CAD build for the part. Positions are in the model's coordinates, mm. Face numbers are marked on the shaded views. A direction names the side the tool comes from. Round coordinates to 2 decimals unless told otherwise and drop trailing zeros. Order: outer loops, then holes, each group sorted by start corner. A loop starts at its lowest first (then second) coordinate and runs counter-clockwise, first axis right, second up.
```python
from build123d import *

# Parameters (mm, degrees)
SKETCH_W        = 165
SKETCH_H        = 45
PAD_DEPTH       = 22
SKETCH001_W     = 133
SKETCH001_H     = 41
POCKET_DEPTH    = 20
SKETCH002_W     = 26
SKETCH002_H     = 41
POCKET001_DEPTH = 20
SKETCH003_W     = 42
SKETCH003_H     = 47
PAD001_DEPTH    = 2
SKETCH008_W     = 42
SKETCH008_H     = 25
PAD002_DEPTH    = 6
SKETCH005_W     = 30
SKETCH005_H     = 13
POCKET002_DEPTH = 8.001
SKETCH009_R     = 1.5
POCKET003_DEPTH = 8.001
SKETCH007_R     = 2.5
POCKET004_DEPTH = 5
SKETCH011_W     = 88.399971
SKETCH011_H     = 21.999902
PAD003_DEPTH    = 2
SKETCH012_W     = 34.60038
SKETCH012_H     = 21.999496
PAD004_DEPTH    = 2


with BuildPart() as part:
    # Sketch → Pad (new body)
    with BuildSketch(Plane.XY):
        with Locations((82.5, 22.5)):
            Rectangle(SKETCH_W, SKETCH_H)
    extrude(amount=PAD_DEPTH)

    # Sketch001 (on Face6 of Pad) → Pocket (cut)
    with BuildSketch(Plane.XY.offset(22)):
        with Locations((68.54825, 22.488898)):
            Rectangle(SKETCH001_W, SKETCH001_H)
    extrude(amount=-POCKET_DEPTH, mode=Mode.SUBTRACT)

    # Sketch002 (on Face5 of Pocket) → Pocket001 (cut)
    with BuildSketch(Plane.XY.offset(22)):
        with Locations((149.979632, 22.458033)):
            Rectangle(SKETCH002_W, SKETCH002_H)
    extrude(amount=-POCKET001_DEPTH, mode=Mode.SUBTRACT)

    # Sketch003 (on Face1 of Pocket001) → Pad001 (join)
    with BuildSketch(Plane(origin=(0, 45, 0), x_dir=(-1, 0, 0), z_dir=(0, 1, 0))):
        with Locations((-55.599999, 23.509954)):
            Rectangle(SKETCH003_W, SKETCH003_H)
    extrude(amount=PAD001_DEPTH)

    # Sketch008 (on Face10 of Pad001) → Pad002 (join)
    with BuildSketch(Plane.XZ.offset(-45)):
        with Locations((55.598549, 34.508675)):
            Rectangle(SKETCH008_W, SKETCH008_H)
    extrude(amount=PAD002_DEPTH)

    # Sketch005 (on Face28 of Pad002) → Pocket002 (cut, through all)
    with BuildSketch(Plane.XZ.offset(-39)):
        with Locations((55.035654, 34.372233)):
            Rectangle(SKETCH005_W, SKETCH005_H)
    extrude(amount=-POCKET002_DEPTH, mode=Mode.SUBTRACT)

    # Sketch009 (on Face32 of Pocket002) → Pocket003 (cut, through all)
    with BuildSketch(Plane.XZ.offset(-39)):
        with Locations((37.021919, 34.390724)):
            Circle(SKETCH009_R)
        with Locations((72.989189, 34.493778)):
            Circle(SKETCH009_R)
    extrude(amount=-POCKET003_DEPTH, mode=Mode.SUBTRACT)

    # Sketch007 (on Face3 of Pocket003) → Pocket004 (cut)
    with BuildSketch(Plane.YZ.offset(165)):
        with Locations((37.952961, 13.56812)):
            Circle(SKETCH007_R)
    extrude(amount=-POCKET004_DEPTH, mode=Mode.SUBTRACT)

    # Sketch011 (on Face2 of Pocket004) → Pad003 (join)
    with BuildSketch(Plane(origin=(0, 45, 0), x_dir=(-1, 0, 0), z_dir=(0, 1, 0))):
        with Locations((-120.799969, 11.000045)):
            Rectangle(SKETCH011_W, SKETCH011_H)
    extrude(amount=PAD003_DEPTH)

    # Sketch012 (on Face2 of Pad003) → Pad004 (join)
    with BuildSketch(Plane(origin=(0, 45, 0), x_dir=(-1, 0, 0), z_dir=(0, 1, 0))):
        with Locations((-17.30019, 10.999748)):
            Rectangle(SKETCH012_W, SKETCH012_H)
    extrude(amount=PAD004_DEPTH)


solid = part.part
```
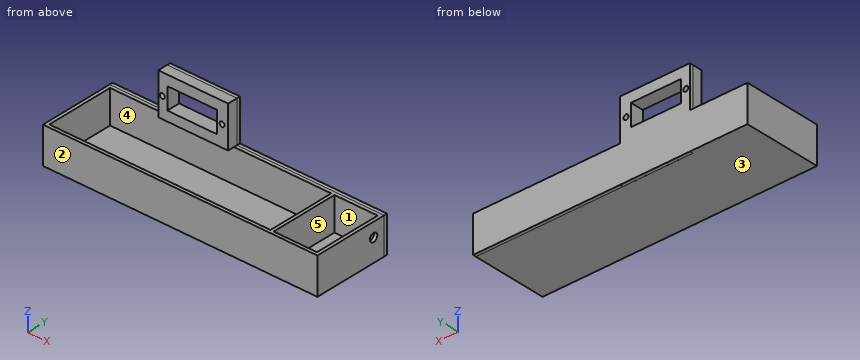
1. Cut at D-D, the plane y = 4. Write the cut outline in (x, z), and give its area (3 significant figures).
2. Cut at A-A, the plane z = 9.5. Give the number of separate pieces and of enclosed holes in the cut face, and give its area (3 significant figures).
3. Cut at C-C, the plane y = 37. Write the cut outline in (x, z).
4. Tool access for the marked faces 1 and 2: list every direction of +Z, -Z, +X, -X, +Y, -Y with a clear straight run to the whole face (end or side of a thin tool).
5. Pin check, flat tips, straight feed: P1, Ø1, axis at y = 46, z = 35, coming from the +X side; P2, Ø5, axis at y = 40.5, z = 33.5, coming from the -X side; P3, Ø20, axis at x = 65, z = 33.5, coming from the -Y side; P4, Ø4, axis at y = 23.5, z = 25, coming from the -X side. Stop position of each tip, or through.
6. Mould opens along Z. For the marked faces 3, 4 and 5 say: released by +Z, released by -Z, zero draft, split by the parting line, or undercut.
7. Drill centre lines: line 1 (X direction, y = 25.5, z = 12); line 2 (Y direction, x = 62, z = 15); line 3 (Z direction, x = 38, y = 40). Where is each one in solid material? Low to high.
Outcome:
1. outline: (0, 0) - (165, 0) - (165, 22) - (162.98, 22) - (162.98, 2) - (136.98, 2) - (136.98, 22) - (135.05, 22) - (135.05, 2) - (2.05, 2) - (2.05, 22) - (0, 22) - close
1. area: 450 mm2
2. separate pieces: 1
2. enclosed holes: 2
2. area: 1,240 mm2
3. outline: (0, 0) - (165, 0) - (165, 11.26) - (162.98, 11.26) - (162.98, 2) - (136.98, 2) - (136.98, 22) - (135.05, 22) - (135.05, 2) - (2.05, 2) - (2.05, 22) - (0, 22) - close; (162.98, 15.88) - (165, 15.88) - (165, 22) - (162.98, 22) - close
4. face 1: +Z
4. face 2: +Z, -Z, +X, -X, -Y
5. P1: stops at x = 76.6
5. P2: stops at x = 34.6
5. P3: stops at y = 39
5. P4: passes through
6. face 3: released by -Z
6. face 4: undercut
6. face 5: zero draft
7. line 1: x = 0 to 2.05, 135.05 to 136.98, 162.98 to 165
7. line 2: y = 0 to 1.99, 42.99 to 47
7. line 3: z = 0 to 2, 22.01 to 33.25, 35.53 to 47.01
